```python
from build123d import *

# Parameters (mm, degrees)
F0_R     = 9.525
F1_DEPTH = 101.6
F2_W     = 9.525
F2_H     = 2.5618169457
F2_W_2   = 8.5228569806
F3_DEPTH = 25.4
F4_R     = 3.175
F5_DEPTH = 25.4
F6_SIZE  = 0.508


with BuildPart() as f1:
    # F0 (on Front) → F1 (new body)
    with BuildSketch(Plane.XZ):
        Circle(F0_R)
    extrude(amount=F1_DEPTH)

    # F2 (on Front) → F3 (cut)
    with BuildSketch(Plane.XZ):
        with Locations((-4.7625, 0)):
            Rectangle(F2_W, F2_H)
        with Locations((4.2614284903, 0)):
            Rectangle(F2_W_2, F2_H)
    extrude(amount=F3_DEPTH, mode=Mode.SUBTRACT)

    # F4 (on face) → F5 (join)
    with BuildSketch(Plane.XZ.offset(101.6)):
        Circle(F4_R)
    extrude(amount=F5_DEPTH)

    # F6
    f6_edges = [f1.edges().sort_by_distance(p)[0] for p in [
        (-3.175, -127, 0),
        (-9.525, -101.6, 0),
        (0.641914, 0, 9.503345),
        (0.641914, 0, -9.503345),
    ]]
    chamfer(f6_edges, length=F6_SIZE)


solid = f1.part
```
The model under review builds one solid part; all positions refer to its coordinate system, in mm. A direction names the side the tool comes from. Coordinates: 2 decimals unless noted, no trailing zeros. Write each loop counter-clockwise with the first axis right and the second up, starting at its lowest first coordinate (ties: lowest second). Pieces come first, ordered by that corner, then holes. Notation, with made-up numbers: (72.25, 27) -> (108.25, 27) arc R8 ccw to (108.25, 34) -> close; hole circle Ø6 at (83, 16). An arc over 180 degrees is marked (long way). One line per item, written item: value. Start each with the question number.
Q1. Add section D-D, the plane y = -8.5. Give the boundary of the cut face in (x, z) (3 decimals).
Q2. Add section A-A, the plane z = 0. Give the boundary of the cut face in (x, y) (3 decimals).
Q3. For faces 1 (the face through (-1, -13, -1.281)), 2 (the face through (4, -101.6, 0)), 3 (the face through (0, -127, 0)), list the 3-axis set-ups (+Z, -Z, +X, -X, +Y, -Y) from which the entire face can be reached by the end or side of a thin tool; tool diameter is ignored.
Q4. Clearance check with flat-ended pins moving along their axes: P1, Ø0.8, axis at y = -7, z = 0, coming from the -X side; P2, Ø2, axis at x = -6.5, z = 0, coming from the +Y side; P3, Ø1, axis at x = -1.5, y = -43, coming from the -Z side. State where each tip first meets the part, or that it passes through.
Q5. Add section B-B, the plane x = 0. Give the boundary of the cut face in (y, z) (3 decimals), then the cut area to 3 significant figures.
Q6. To check wall thickness, follow probe 1 along Y at (x, z) = (6.75, 4); probe 2 along Z at (x, y) = (0.25, -51); probe 3 along Z at (x, y) = (1, -4.5). State the ranges of each line that lie inside material, in increasing order.
Q7. Add section C-C, the plane y = -105. Give the boundary of the cut face in (x, z) (3 decimals), then the cut area to 3 significant figures.
Response:
1. outline: (-9.438, -1.281) arc R9.525 ccw (long way) to (-9.438, 1.281) -> (8.523, 1.281) -> (8.523, -1.281) -> close
2. outline: (-9.525, -101.092) -> (-9.017, -101.6) -> (-3.175, -101.6) -> (-3.175, -126.492) -> (-2.667, -127) -> (2.667, -127) -> (3.175, -126.492) -> (3.175, -101.6) -> (9.017, -101.6) -> (9.525, -101.092) -> (9.525, -0.508) -> (9.017, 0) -> (8.523, 0) -> (8.523, -25.4) -> (-9.525, -25.4) -> close
3. face 1: -X, +Y
3. face 2: -Y
3. face 3: +Z, -Z, +X, -X, -Y
4. P1: x = 8.52
4. P2: y = -25.4
4. P3: z = -9.47
5. outline: (-127, -2.667) -> (-126.492, -3.175) -> (-101.6, -3.175) -> (-101.6, -9.017) -> (-101.092, -9.525) -> (-0.508, -9.525) -> (0, -9.017) -> (0, -1.281) -> (-25.4, -1.281) -> (-25.4, 1.281) -> (0, 1.281) -> (0, 9.017) -> (-0.508, 9.525) -> (-101.092, 9.525) -> (-101.6, 9.017) -> (-101.6, 3.175) -> (-126.492, 3.175) -> (-127, 2.667) -> close
5. area: 2,030 mm²
6. probe 1: -101.6 to 0
6. probe 2: -9.52 to 9.52
6. probe 3: -9.47 to -1.28, 1.28 to 9.47
7. outline: circle Ø6.35 at (0, 0)
7. area: 31.7 mm²
